Check sheet for the modelled part. Datum: model origin and axes. Units: mm. A direction names the side the tool comes from. Coordinates: 2 decimals unless noted, no trailing zeros. Order: outer loops, then holes, each group sorted by start corner. A loop starts at its lowest first (then second) coordinate and runs counter-clockwise, first axis right, second up.
from build123d import *

# Parameters (mm, degrees)
SKETCH_1_W           = 94
SKETCH_1_H           = 30
EXTRUDE_2_DEPTH      = 120
SKETCH_2_W           = 84
SKETCH_2_H           = 110
CUT_EXTRUDE_1_DEPTH  = 20
SKETCH_4_W           = 12.8042226
SKETCH_4_H           = 20
CUT_EXTRUDE_5_DEPTH  = 20
SKETCH_9_W           = 17.034378807
SKETCH_9_H           = 15
CUT_EXTRUDE_6_DEPTH  = 20
SKETCH_10_W          = 26
SKETCH_10_H          = 34
EXTRUDE_2_2_DEPTH    = 26
SKETCH_16_R          = 11.5
CUT_EXTRUDE_8_DEPTH  = 126.231871204
FILLET_2_R           = 10
FILLET_3_R           = 10
FILLET_4_R           = 10
SKETCH_20_R          = 1.5
CUT_EXTRUDE_12_DEPTH = 10
SKETCH_21_W          = 28.864787598
SKETCH_21_H          = 27.787348415
CUT_EXTRUDE_13_DEPTH = 40
CUT_EXTRUDE_START    = -50
SKETCH_22_W          = 124.707119116
SKETCH_22_H          = 18.117072108
CUT_EXTRUDE_14_DEPTH = 150
SKETCH_23_R          = 1.4
EXTRUDE_4_DEPTH      = 8
SKETCH_25_W          = 5
SKETCH_25_H          = 5
CUT_EXTRUDE_15_DEPTH = 4.45
SKETCH_28_W          = 5
SKETCH_28_H          = 5
EXTRUDE_5_DEPTH      = 4.45


with BuildPart() as part:
    # 스케치1 → Extrude 2 (new body)
    with BuildSketch(Plane.XY):
        with Locations((47, 15)):
            Rectangle(SKETCH_1_W, SKETCH_1_H)
    extrude(amount=EXTRUDE_2_DEPTH)

    # 스케치2 → 컷-돌출1 (cut)
    with BuildSketch(Plane(origin=(0, 30, 0), x_dir=(1, 0, 0), z_dir=(0, 1, 0))):
        with Locations((47, -60)):
            Rectangle(SKETCH_2_W, SKETCH_2_H)
    extrude(amount=-CUT_EXTRUDE_1_DEPTH, mode=Mode.SUBTRACT)

    # 스케치4 → 컷-돌출5 (cut)
    with BuildSketch(Plane(origin=(0, 30, 0), x_dir=(1, 0, 0), z_dir=(0, 1, 0))):
        with Locations((95.4021113, -94)):
            Rectangle(SKETCH_4_W, SKETCH_4_H)
    extrude(amount=-CUT_EXTRUDE_5_DEPTH, mode=Mode.SUBTRACT)

    # 스케치9 → 컷-돌출6 (cut)
    with BuildSketch(Plane(origin=(0, 30, 0), x_dir=(1, 0, 0), z_dir=(0, 1, 0))):
        with Locations((97.517189403, -22.5)):
            Rectangle(SKETCH_9_W, SKETCH_9_H)
    extrude(amount=-CUT_EXTRUDE_6_DEPTH, mode=Mode.SUBTRACT)

    # 스케치10 → Extrude 2 2 (add)
    with BuildSketch(Plane(origin=(0, 0, 0), x_dir=(-1, 0, 0), z_dir=(0, -1, 0))):
        with Locations((-47, -59.883065639)):
            Rectangle(SKETCH_10_W, SKETCH_10_H)
    extrude(amount=EXTRUDE_2_2_DEPTH)

    # 스케치16 → 컷-돌출8 (cut, through all)
    with BuildSketch(Plane(origin=(0, 0, 42.883065639), x_dir=(-1, 0, 0), z_dir=(0, 0, -1))):
        with Locations((-47, -13)):
            Circle(SKETCH_16_R)
    extrude(amount=-CUT_EXTRUDE_8_DEPTH, mode=Mode.SUBTRACT)

    # 필렛2
    fillet_2_edges = [part.edges().sort_by_distance(p)[0] for p in [
        (0, 15, 0),
    ]]
    fillet(fillet_2_edges, radius=FILLET_2_R)

    # 필렛3
    fillet_3_edges = [part.edges().sort_by_distance(p)[0] for p in [
        (94, 15, 120),
        (0, 15, 120),
        (94, 15, 0),
    ]]
    fillet(fillet_3_edges, radius=FILLET_3_R)

    # 필렛4
    fillet_4_edges = [part.edges().sort_by_distance(p)[0] for p in [
        (47, 0, 0),
        (2.928932188, 0, 2.928932188),
        (0, 0, 60),
        (47, 0, 120),
        (94, 0, 60),
        (91.071067812, 0, 2.928932188),
        (91.071067812, 0, 117.071067812),
        (2.928932188, 0, 117.071067812),
    ]]
    fillet(fillet_4_edges, radius=FILLET_4_R - 0.0001)  # a hair under: the kernel refuses the full size

    # 스케치20 → 컷-돌출12 (cut)
    with BuildSketch(Plane(origin=(0, 30, 0), x_dir=(1, 0, 0), z_dir=(0, 1, 0))):
        with Locations(Location((25.192810861, -2.5, 0), (0, 0, 270))):
            Circle(SKETCH_20_R)
        with Locations(Location((68.807189139, -2.5, 0), (0, 0, 90))):
            Circle(SKETCH_20_R)
        with Locations(Location((25.192810861, -117.5, 0), (0, 0, 270))):
            Circle(SKETCH_20_R)
        with Locations(Location((68.807189139, -117.5, 0), (0, 0, 90))):
            Circle(SKETCH_20_R)
    extrude(amount=-CUT_EXTRUDE_12_DEPTH, mode=Mode.SUBTRACT)

    # 스케치21 → 컷-돌출13 (cut)
    with BuildSketch(Plane.XY.offset(76.883065639)):
        with Locations((48.432393799, -13.893674208)):
            Rectangle(SKETCH_21_W, SKETCH_21_H)
    extrude(amount=-CUT_EXTRUDE_13_DEPTH, mode=Mode.SUBTRACT)

    # 스케치22 → 컷-돌출14 (cut)
    with BuildSketch(Plane(origin=(5, 0, 0), x_dir=(0, 0, -1), z_dir=(1, 0, 0)).offset(CUT_EXTRUDE_START)):
        with Locations((-62.353559558, 23.504988421)):
            Rectangle(SKETCH_22_W, SKETCH_22_H)
    extrude(amount=CUT_EXTRUDE_14_DEPTH, mode=Mode.SUBTRACT)

    # 스케치23 → 보스-돌출4 (add)
    with BuildSketch(Plane(origin=(0, 14.446452367, 0), x_dir=(1, 0, 0), z_dir=(0, 1, 0))):
        with Locations(Location((25.192810861, -117.5, 0), (0, 0, 270))):
            Circle(SKETCH_23_R)
        with Locations(Location((68.807189139, -117.5, 0), (0, 0, 90))):
            Circle(SKETCH_23_R)
        with Locations(Location((25.192810861, -2.5, 0), (0, 0, 270))):
            Circle(SKETCH_23_R)
        with Locations(Location((68.807189139, -2.5, 0), (0, 0, 90))):
            Circle(SKETCH_23_R)
    extrude(amount=EXTRUDE_4_DEPTH)

    # 스케치25 → 컷-돌출15 (cut)
    with BuildSketch(Plane(origin=(0, 14.446452367, 0), x_dir=(1, 0, 0), z_dir=(0, 1, 0))):
        with Locations((91.5, -32.5)):
            Rectangle(SKETCH_25_W, SKETCH_25_H)
    extrude(amount=-CUT_EXTRUDE_15_DEPTH, mode=Mode.SUBTRACT)

    # 스케치28 → 보스-돌출5 (add)
    with BuildSketch(Plane(origin=(0, 14.446452367, 0), x_dir=(1, 0, 0), z_dir=(0, 1, 0))):
        with Locations((91.5, -86.5)):
            Rectangle(SKETCH_28_W, SKETCH_28_H)
    extrude(amount=-EXTRUDE_5_DEPTH)


solid = part.part
(1) Go/stop test with flat-tipped pins: P1, Ø6, axis at x = 33, y = 15.5, coming from the -Z side; P2, Ø4, axis at y = 5.5, z = 107, coming from the -X side; P3, Ø1.3, axis at x = 91, y = 12.5, coming from the -Z side; P4, Ø4, axis at x = 92.5, z = 68.5, coming from the +Y side. Record where each tip stops, or that it passes through.
Filled in:
P1: stops at z = 0
P2: stops at x = 0.32
P3: stops at z = 2.27
P4: stops at y = 14.45
(2) Tool access check on faces 4 (the flat face through (89, 12, 10)), 5 (the cylindrical face through (90.99, 12.25, 117.15)), 6 (the flat face through (91, 12, 35)). Record the directions out of +Z, -Z, +X, -X, +Y, -Y that give a thin tool (end or side, any length) a straight path to the whole face; none if there is none.
Filled in:
face 4: +Y
face 5: +Z, +X, +Y, -Y
face 6: +X, +Y
(3) Cross-section at C-C (x = 11.5). Enter the section's corners in (y, z).
Filled in:
outline: (0, 10) arc R10 ccw to (10, 0) - (14.45, 0) - (14.45, 5) - (10, 5) - (10, 115) - (14.45, 115) - (14.45, 120) - (10, 120) arc R10 ccw to (0, 110) - close
(4) Thickness scan on probe 1 along Z at (x, y) = (51.5, 10.25); probe 2 along X at (y, z) = (11, 65); probe 3 along Y at (x, z) = (41, 82.5). Record the ranges inside material, lowest first.
Filled in:
probe 1: z = 0 to 5, 115 to 120
probe 2: x = 0 to 5, 89 to 94
probe 3: y = 0 to 10
(5) Release check for a two-part mould opening along Z. For faces 1 (the cylindrical face through (69.66, 18.39, 118.61)), 2 (the cylindrical face through (3.01, 2.85, 59.3)), 3 (the cylindrical face through (47.52, 2.85, 3.01)) record: +Z half, -Z half, draft (parallel to the pull), parting line (faces both ways), or undercut.
Filled in:
face 1: undercut
face 2: draft
face 3: -Z half
(6) Cross-section at B-B (z = 72). Enter the section's corners in (x, y), and give its area (3 significant figures).
Filled in:
outline: (0, 10) arc R10 ccw to (10, 0) - (84, 0) arc R10 ccw to (94, 10) - (94, 14.45) - (89, 14.45) - (89, 10) - (5, 10) - (5, 14.45) - (0, 14.45) - close
area: 942 mm2
(7) Cross-section at A-A (y = 11.5). Enter the section's corners in (x, z), and give its area (3 significant figures).
Filled in:
outline: (0, 10) arc R10 ccw to (10, 0) - (84, 0) arc R10 ccw to (94, 10) - (94, 15) - (89, 15) - (89, 5) - (5, 5) - (5, 115) - (89, 115) - (89, 104) - (94, 104) - (94, 110) arc R10 ccw to (84, 120) - (10, 120) arc R10 ccw to (0, 110) - close; (89, 35) - (94, 35) - (94, 89) - (89, 89) - close
area: 1,780 mm2
